For this review, take the finished solid that the model builds, in its own axes (mm). Face numbers are marked on the shaded views. A direction names the side the tool comes from. Give positions to 0.01 mm unless a question says otherwise; leave off trailing zeros. Loops run counter-clockwise (first coordinate to the right, second up) from the corner with the lowest first, then second, coordinate; pieces in that order, holes last.
```python
from build123d import *

# Parameters (mm, degrees)
BOSS_EXTRUDE1_DEPTH = 9
SKETCH2_R           = 2
CUT_EXTRUDE1_DEPTH  = 9
BOSS_EXTRUDE2_DEPTH = 9
SKETCH5_W           = 47
SKETCH5_H           = 2.614456703
BOSS_EXTRUDE3_DEPTH = 4
FILLET1_R           = 2
FILLET4_R           = 2
BOSS_EXTRUDE5_DEPTH = 5
FILLET5_R           = 2


with BuildPart() as part:
    # Sketch1 → Boss-Extrude1 (new body)
    with BuildSketch(Plane.XY):
        Polygon((0, 0), (10, 0), (10, -18), (37, -18), (37, 0), (47, 0), (47, -2.614456703), (41, -2.614456703), (41, -21), (6, -21), (6, -2.614456703), (0, -2.614456703), align=None)
    extrude(amount=BOSS_EXTRUDE1_DEPTH)

    # Sketch2 → Cut-Extrude1 (cut)
    with BuildSketch(Plane.XZ.offset(2.614456703)):
        with Locations((3, 4.5)):
            Circle(SKETCH2_R)
    cut_extrude1 = extrude(amount=-CUT_EXTRUDE1_DEPTH, mode=Mode.SUBTRACT)

    # Mirror1: Cut-Extrude1 across plane
    add(cut_extrude1.mirror(Plane(origin=(23.5, 0, 0), x_dir=(0, 0, 1), z_dir=(1, 0, 0))), mode=Mode.SUBTRACT)

    # Sketch3 → Boss-Extrude2 (add)
    with BuildSketch(Plane.XY.offset(9)):
        Polygon((0, 0), (0, -2.614456703), (6, -2.614456703), (6, -21), (41, -21), (41, -2.614456703), (47, -2.614456703), (47, 0), (37, 0), (37, -18), (10, -18), (10, 0), align=None)
    extrude(amount=BOSS_EXTRUDE2_DEPTH)

    # Sketch5 → Boss-Extrude3 (add)
    with BuildSketch(Plane.XY.offset(18)):
        with Locations((23.5, -1.307228352)):
            Rectangle(SKETCH5_W, SKETCH5_H)
    extrude(amount=BOSS_EXTRUDE3_DEPTH)

    # Fillet1
    fillet1_edges = [part.edges().sort_by_distance(p)[0] for p in [
        (0, -1.307228352, 22),
        (47, -1.307228352, 22),
    ]]
    fillet(fillet1_edges, radius=FILLET1_R)

    # Fillet4
    fillet4_edges = [part.edges().sort_by_distance(p)[0] for p in [
        (47, -1.307228352, 0),
        (0, -1.307228352, 0),
        (41, -21, 9),
        (6, -21, 9),
    ]]
    fillet(fillet4_edges, radius=FILLET4_R)

    # Sketch9 → Boss-Extrude5 (add)
    with BuildSketch(Plane.XZ.offset(2.614456703)):
        Polygon((6, 22), (6, 18), (10, 18), (37, 18), (41, 18), (41, 22), align=None)
    extrude(amount=BOSS_EXTRUDE5_DEPTH)

    # Fillet5
    fillet5_edges = [part.edges().sort_by_distance(p)[0] for p in [
        (23.5, -7.614456703, 22),
    ]]
    fillet(fillet5_edges, radius=FILLET5_R)


solid = part.part
```
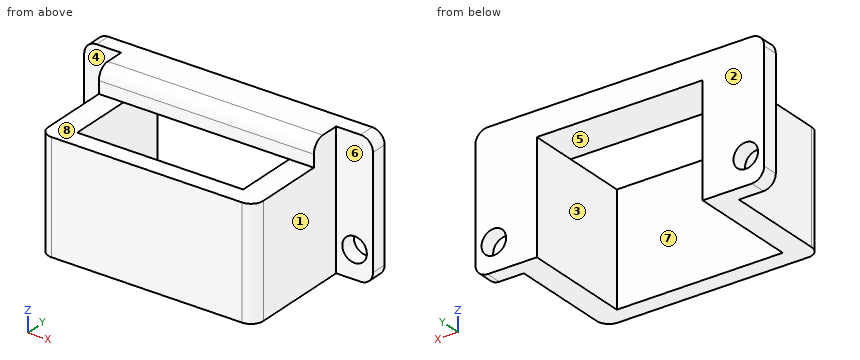
Q1. Machinability: for the marked faces 4, 5, 6, 7 and 8, which of the approach directions +Z, -Z, +X, -X, +Y, -Y give a long, thin tool a straight path to every point of the face, cutting with its end or side? Answer none if there is none.
Answers:
face 4: +Z, -Z, -X, -Y
face 5: -Z, +Y
face 6: +Z, -Z, +X, -Y
face 7: +Z, -Z, +Y
face 8: +Z, +X, -X, -Y
Q2. Mouldability with a two-part tool opening along X and no side actions: class the marked faces 1, 2 and 3 as +X half, -X half, draft (parallel to the pull), parting line (faces both ways), or undercut.
Answers:
face 1: +X half
face 2: draft
face 3: undercut
Q3. For pin 1 Ø5 at (y, z) = (-18.5, 11.5) entering from +X; pin 2 Ø6.5 at (x, z) = (4, 15.5) entering from -Y; pin 3 Ø2 at (x, y) = (40.5, -8) entering from +Z, all flat-tipped, find the tip position at first contact; note any pin that passes through.
Answers:
pin 1: stops at x = 41
pin 2: stops at y = -20.85
pin 3: stops at z = 21.44
Q4. Consider section D-D on y = -4. Give the boundary of the cut face in (x, z).
Answers:
outline: (6, 0) - (10, 0) - (10, 18) - (37, 18) - (37, 0) - (41, 0) - (41, 22) - (6, 22) - close
Q5. For probe 1 along X at (y, z) = (-11, 14.75); probe 2 along Z at (x, y) = (3, -1.5); probe 3 along Y at (x, z) = (7.5, 20), list the stretches that pass through material, from the lowest coordinate up.
Answers:
probe 1: x = 6 to 10, 37 to 41
probe 2: z = 0 to 2.5, 6.5 to 22
probe 3: y = -7.61 to 0
Q6. Consider section C-C on z = 4.5. Give the boundary of the cut face in (x, y).
Answers:
outline: (0, -2.61) - (1, -2.61) - (1, 0) - (0, 0) - close; (5, -2.61) - (6, -2.61) - (6, -19) arc R2 ccw to (8, -21) - (39, -21) arc R2 ccw to (41, -19) - (41, -2.61) - (42, -2.61) - (42, 0) - (37, 0) - (37, -18) - (10, -18) - (10, 0) - (5, 0) - close; (46, -2.61) - (47, -2.61) - (47, 0) - (46, 0) - close
Q7. Consider section A-A on x = 12.5. Give the boundary of the cut face in (y, z).
Answers:
outline: (-21, 0) - (-18, 0) - (-18, 18) - (-21, 18) - close; (-7.61, 18) - (0, 18) - (0, 22) - (-5.61, 22) arc R2 ccw to (-7.61, 20) - close
Q8. Consider section B-B on y = -10. Give the boundary of the cut face in (x, z), plus the area to 3 significant figures.
Answers:
outline: (6, 0) - (10, 0) - (10, 18) - (6, 18) - close; (37, 0) - (41, 0) - (41, 18) - (37, 18) - close
area: 144 mm2
